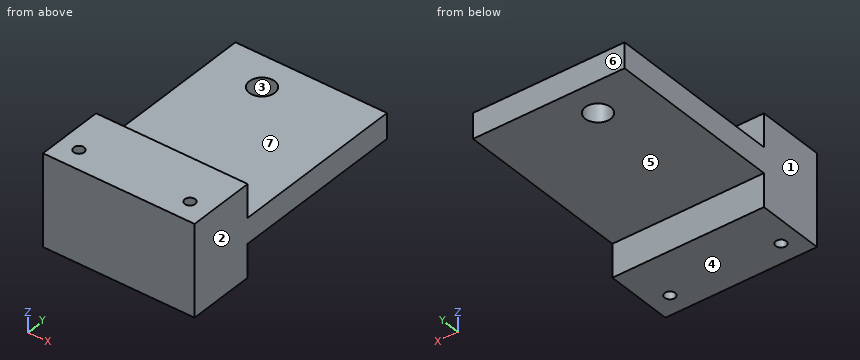
from build123d import *

# Parameters (mm, degrees)
SIDE_W                                      = 35.95
SIDE_H                                      = 10
AUFSATZ_LINEAR_AUSTRAGEN1_DEPTH             = 10.85
AUFSATZ_LINEAR_AUSTRAGEN1_DEPTH_BACK        = 10.85
SKIZZE5_R                                   = 1.25
SCHNITT_LINEAR_AUSTRAGEN1_DEPTH             = 11.85
SCHNITT_LINEAR_AUSTRAGEN1_DEPTH_BACK        = 11.85
TOPEXTENSION_W                              = 35.95
TOPEXTENSION_H                              = 48
TOPEXTENSION_R                              = 3
AUFSATZ_LINEAR_AUSTRAGEN2_DEPTH             = 3
AUFSATZ_LINEAR_AUSTRAGEN2_DEPTH_BACK        = 3
AUFSATZ_LINEAR_AUSTRAGEN3_REACH             = 12.85
SKIZZE8_W                                   = 35.95
SKIZZE8_H                                   = 6
AUFSATZ_LINEAR_AUSTRAGEN3_DIRECTION_2_REACH = 12.85


with BuildPart() as part:
    # Side → Aufsatz-Linear austragen1 (new body, two sides)
    with BuildSketch(Plane.XY) as aufsatz_linear_austragen1_sk:
        with Locations((5.375, 625)):
            Rectangle(SIDE_W, SIDE_H)
    extrude(amount=AUFSATZ_LINEAR_AUSTRAGEN1_DEPTH)
    extrude(aufsatz_linear_austragen1_sk.sketch, amount=-AUFSATZ_LINEAR_AUSTRAGEN1_DEPTH_BACK)

    # Skizze5 → Schnitt-Linear austragen1 (cut, two sides)
    with BuildSketch(Plane.XY) as schnitt_linear_austragen1_sk:
        with Locations((-8, 625)):
            Circle(SKIZZE5_R)
        with Locations((18.35, 625)):
            Circle(SKIZZE5_R)
    extrude(amount=SCHNITT_LINEAR_AUSTRAGEN1_DEPTH, mode=Mode.SUBTRACT)
    extrude(schnitt_linear_austragen1_sk.sketch, amount=-SCHNITT_LINEAR_AUSTRAGEN1_DEPTH_BACK, mode=Mode.SUBTRACT)

    # TopExtension → Aufsatz-Linear austragen2 (add, two sides)
    with BuildSketch(Plane.XY) as aufsatz_linear_austragen2_sk:
        with Locations((5.375, 654)):
            Rectangle(TOPEXTENSION_W, TOPEXTENSION_H)
        with Locations((0, 670)):
            Circle(TOPEXTENSION_R, mode=Mode.SUBTRACT)
    extrude(amount=AUFSATZ_LINEAR_AUSTRAGEN2_DEPTH)
    extrude(aufsatz_linear_austragen2_sk.sketch, amount=-AUFSATZ_LINEAR_AUSTRAGEN2_DEPTH_BACK)

    # Aufsatz-Linear austragen3: up to this face of the body (flat: up to its plane)
    aufsatz_linear_austragen3_end = Plane(part.part.faces().sort_by_distance((5.38061508, 625, 10.85))[0])
    # Skizze8 → Aufsatz-Linear austragen3 (add, up to the picked face)
    with BuildSketch(Plane.XY, mode=Mode.PRIVATE) as aufsatz_linear_austragen3_sk1:
        with Locations((5.375, 633)):
            Rectangle(SKIZZE8_W, SKIZZE8_H)
    aufsatz_linear_austragen3_tool1 = split(extrude(aufsatz_linear_austragen3_sk1.sketch, amount=AUFSATZ_LINEAR_AUSTRAGEN3_REACH, mode=Mode.PRIVATE), bisect_by=aufsatz_linear_austragen3_end, keep=Keep.BOTH, mode=Mode.PRIVATE)
    add(aufsatz_linear_austragen3_tool1.solids().sort_by_distance((5.375, 633, 0))[0])

    # Aufsatz-Linear austragen3 direction 2: up to this face of the body (flat: up to its plane)
    aufsatz_linear_austragen3_direction_2_end = Plane(part.part.faces().sort_by_distance((5.38061508, 625, -10.85))[0])
    # Skizze8 → Aufsatz-Linear austragen3 direction 2 (add, up to the picked face)
    with BuildSketch(Plane.XY, mode=Mode.PRIVATE) as aufsatz_linear_austragen3_direction_2_sk1:
        with Locations((5.375, 633)):
            Rectangle(SKIZZE8_W, SKIZZE8_H)
    aufsatz_linear_austragen3_direction_2_tool1 = split(extrude(aufsatz_linear_austragen3_direction_2_sk1.sketch, amount=-AUFSATZ_LINEAR_AUSTRAGEN3_DIRECTION_2_REACH, mode=Mode.PRIVATE), bisect_by=aufsatz_linear_austragen3_direction_2_end, keep=Keep.BOTH, mode=Mode.PRIVATE)
    add(aufsatz_linear_austragen3_direction_2_tool1.solids().sort_by_distance((5.375, 633, 0))[0])


solid = part.part
Here's how the part is built. I have some questions about the finished solid (model axes, mm). Face numbers are marked on the shaded views. A direction names the side the tool comes from. Give positions to 0.01 mm unless a question says otherwise; leave off trailing zeros. Order: outer loops, then holes, each group sorted by start corner. A loop starts at its lowest first (then second) coordinate and runs counter-clockwise, first axis right, second up. Notation, with made-up numbers: (-27, 56) -> (6, 56) arc R32 cw to (6, 82) -> close; hole circle Ø7 at (0.5, -1.5). An arc over 180 degrees is marked (long way). Use a Markdown table: item, result. Add a question column.
Item 1: Imagine slicing it at C-C on y = 670. Please give me the cut outline in (x, z), plus the area to 3 significant figures.
Item 2: Will these pins go through, and if not, where does the flat tip stop? pin 1 (3 mm diameter, centred on x = 17.5, z = -5.5, fed in from +Y); pin 2 (11 mm diameter, centred on x = 4.5, y = 664.5, fed in from -Z).
Item 3: Imagine slicing it at A-A on x = -8. Please give me the cut outline in (y, z).
Item 4: For the marked faces 5, 6 and 7, which set-ups out of +Z, -Z, +X, -X, +Y, -Y let a thin tool reach every point of the face, with its end or its side?
Item 5: I need wall thicknesses on line 1 (X direction, y = 625, z = 6); line 2 (Y direction, x = 18.35, z = -2.5); line 3 (Y direction, x = -8, z = 3.5). Which ranges of each line are inside material? Lowest first, please.
Item 6: Imagine slicing it at D-D on z = -2.25. Please give me the cut outline in (x, y).
Item 7: If we mould it in two halves opening along X, with no side actions, what happens to the marked faces 1, 2, 3 and 4? For each: pulls with the +X half, pulls with the -X half, needs draft (parallel to the pull), parting line crosses it, or undercut.
Item 8: Imagine slicing it at B-B on y = 625. Please give me the cut outline in (x, z), plus the area to 3 significant figures.
Data:
| question | item | result |
|---|---|---|
| 1 | outline | (-12.6, -3) -> (-3, -3) -> (-3, 3) -> (-12.6, 3) -> close; (3, -3) -> (23.35, -3) -> (23.35, 3) -> (3, 3) -> close |
| 1 | area | 180 mm² |
| 2 | pin 1 | stops at y = 636 |
| 2 | pin 2 | stops at z = -3 |
| 3 | outline | (620, -10.85) -> (623.75, -10.85) -> (623.75, 10.85) -> (620, 10.85) -> close; (626.25, -10.85) -> (636, -10.85) -> (636, -3) -> (678, -3) -> (678, 3) -> (636, 3) -> (636, 10.85) -> (626.25, 10.85) -> close |
| 4 | face 5 | -Z, +X, -X, +Y |
| 4 | face 6 | +Z, -Z, +X, -X, +Y |
| 4 | face 7 | +Z, +X, -X, +Y |
| 5 | line 1 | x = -12.6 to -9.25, -6.75 to 17.1, 19.6 to 23.35 |
| 5 | line 2 | y = 620 to 623.75, 626.25 to 678 |
| 5 | line 3 | y = 620 to 623.75, 626.25 to 636 |
| 6 | outline | (-12.6, 620) -> (23.35, 620) -> (23.35, 678) -> (-12.6, 678) -> close; hole circle Ø2.5 at (-8, 625); hole circle Ø6 at (0, 670); hole circle Ø2.5 at (18.35, 625) |
| 7 | face 1 | pulls with the -X half |
| 7 | face 2 | pulls with the +X half |
| 7 | face 3 | undercut |
| 7 | face 4 | needs draft |
| 8 | outline | (-12.6, -10.85) -> (-9.25, -10.85) -> (-9.25, 10.85) -> (-12.6, 10.85) -> close; (-6.75, -10.85) -> (17.1, -10.85) -> (17.1, 10.85) -> (-6.75, 10.85) -> close; (19.6, -10.85) -> (23.35, -10.85) -> (23.35, 10.85) -> (19.6, 10.85) -> close |
| 8 | area | 672 mm² |
